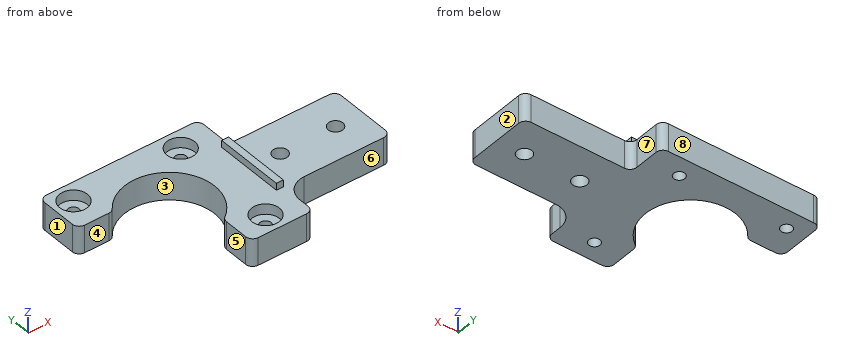
from build123d import *

# Parameters (mm, degrees)
ESQUISSE1_W             = 77
ESQUISSE1_H             = 42
BOSS_EXTRU_1_DEPTH      = 8
ESQUISSE3_R             = 4
ENL_V_MAT_EXTRU_1_DEPTH = 3
ESQUISSE4_R             = 13
ENL_V_MAT_EXTRU_2_DEPTH = 9
ESQUISSE5_W             = 28
ESQUISSE5_H             = 28
ENL_V_MAT_EXTRU_3_DEPTH = 9
ESQUISSE10_R            = 1.6
ENL_V_MAT_EXTRU_4_DEPTH = 6
ESQUISSE11_W            = 31
ESQUISSE11_H            = 11
ENL_V_MAT_EXTRU_5_DEPTH = 9
ESQUISSE12_R            = 2.1
ENL_V_MAT_EXTRU_6_DEPTH = 9
CONG_1_R                = 6
CONG_2_R                = 2
SKETCH1_W               = 2
SKETCH1_H               = 20
BOSS_EXTRUDE1_DEPTH     = 2


with BuildPart() as part:
    # Esquisse1 → Boss.-Extru.1 (new body)
    with BuildSketch(Plane.XY):
        with Locations((38.5, 21)):
            Rectangle(ESQUISSE1_W, ESQUISSE1_H)
    extrude(amount=BOSS_EXTRU_1_DEPTH)

    # Esquisse3 → Enlèv. mat.-Extru.1 (cut)
    with BuildSketch(Plane.XY.offset(8)):
        with Locations((5.5, 36.5)):
            Circle(ESQUISSE3_R)
        with Locations((36.5, 36.5)):
            Circle(ESQUISSE3_R)
        with Locations((36.5, 5.5)):
            Circle(ESQUISSE3_R)
    extrude(amount=-ENL_V_MAT_EXTRU_1_DEPTH, mode=Mode.SUBTRACT)

    # Esquisse4 → Enlèv. mat.-Extru.2 (cut, through all)
    with BuildSketch(Plane.XY.offset(8)):
        with Locations((21, 21)):
            Circle(ESQUISSE4_R)
    extrude(amount=-ENL_V_MAT_EXTRU_2_DEPTH, mode=Mode.SUBTRACT)

    # Esquisse5 → Enlèv. mat.-Extru.3 (cut, through all)
    with BuildSketch(Plane.XY.offset(8)):
        with Locations((14, 14)):
            Rectangle(ESQUISSE5_W, ESQUISSE5_H)
    extrude(amount=-ENL_V_MAT_EXTRU_3_DEPTH, mode=Mode.SUBTRACT)

    # Esquisse10 → Enlèv. mat.-Extru.4 (cut, through all)
    with BuildSketch(Plane.XY.offset(5)):
        with Locations((5.5, 36.5)):
            Circle(ESQUISSE10_R)
        with Locations((36.5, 36.5)):
            Circle(ESQUISSE10_R)
        with Locations((36.5, 5.5)):
            Circle(ESQUISSE10_R)
    extrude(amount=-ENL_V_MAT_EXTRU_4_DEPTH, mode=Mode.SUBTRACT)

    # Esquisse11 → Enlèv. mat.-Extru.5 (cut, through all)
    with BuildSketch(Plane.XY.offset(8)):
        with Locations((61.5, 5.5)):
            Rectangle(ESQUISSE11_W, ESQUISSE11_H)
        with Locations((61.5, 36.5)):
            Rectangle(ESQUISSE11_W, ESQUISSE11_H)
    extrude(amount=-ENL_V_MAT_EXTRU_5_DEPTH, mode=Mode.SUBTRACT)

    # Esquisse12 → Enlèv. mat.-Extru.6 (cut, through all)
    with BuildSketch(Plane.XY.offset(8)):
        with Locations((53, 21)):
            Circle(ESQUISSE12_R)
        with Locations((69, 21)):
            Circle(ESQUISSE12_R)
    extrude(amount=-ENL_V_MAT_EXTRU_6_DEPTH, mode=Mode.SUBTRACT)

    # Congé1
    cong_1_edges = [part.edges().sort_by_distance(p)[0] for p in [
        (46, 11, 4),
    ]]
    fillet(cong_1_edges, radius=CONG_1_R)

    # Congé2
    cong_2_edges = [part.edges().sort_by_distance(p)[0] for p in [
        (28, 10.04554885, 4),
        (10.04554885, 28, 4),
        (0, 28, 4),
        (28, 0, 4),
        (77, 11, 4),
        (46, 0, 4),
        (0, 42, 4),
        (77, 31, 4),
        (46, 31, 4),
        (46, 42, 4),
    ]]
    fillet(cong_2_edges, radius=CONG_2_R)

    # Sketch1 → Boss-Extrude1 (add)
    with BuildSketch(Plane.XY.offset(8)):
        with Locations((45, 21)):
            Rectangle(SKETCH1_W, SKETCH1_H)
    extrude(amount=BOSS_EXTRUDE1_DEPTH)


solid = part.part
Can you work these out from the model? Positions are in its coordinate system, mm. Face numbers are marked on the shaded views. A direction names the side the tool comes from. Coordinates: 2 decimals unless noted, no trailing zeros. Order: outer loops, then holes, each group sorted by start corner. A loop starts at its lowest first (then second) coordinate and runs counter-clockwise, first axis right, second up. Notation, with made-up numbers: M -3,13 L 12,13 A16 ccw 12,26 Z; hole C 56.5,71.25 d11. An arc over 180 degrees is marked long. Write item = value, one per line.
(1) If we mould it in two halves opening along X, with no side actions, what happens to the marked faces 1, 2, 3 and 4? For each: pulls with the +X half, pulls with the -X half, needs draft (parallel to the pull), parting line crosses it, or undercut.
Results are:
face_1 = pulls with the -X half
face_2 = pulls with the +X half
face_3 = undercut
face_4 = needs draft
(2) For pin 1 Ø3.5 at (y, z) = (3, 5) entering from +X; pin 2 Ø6 at (y, z) = (4.5, 7.5) entering from +X; pin 3 Ø23.5 at (x, y) = (21, 21) entering from +Z; pin 4 Ø5.5 at (y, z) = (6, 5.5) entering from -X, each with a flat end and sliding along its axis, tell me the tip position at first contact or that it passes through.
Results are:
pin_1 = 46
pin_2 = 46.55
pin_3 = through
pin_4 = 28
(3) Suppose I cut it at B-B on x = 69. Please give me the cut outline in (y, z).
Results are:
outline = M 11,0 L 18.9,0 L 18.9,8 L 11,8 Z; M 23.1,0 L 31,0 L 31,8 L 23.1,8 Z
(4) Suppose I cut it at A-A on y = 36.5. Please give me the cut outline in (x, z).
Results are:
outline = M 0,0 L 3.9,0 L 3.9,5 L 1.5,5 L 1.5,8 L 0,8 Z; M 7.1,0 L 34.9,0 L 34.9,5 L 32.5,5 L 32.5,8 L 9.5,8 L 9.5,5 L 7.1,5 Z; M 38.1,0 L 46,0 L 46,8 L 40.5,8 L 40.5,5 L 38.1,5 Z
(5) Suppose I cut it at D-D on x = 36.5. Please give me the cut outline in (y, z), plus the area to 3 significant figures.
Results are:
outline = M 0,0 L 3.9,0 L 3.9,5 L 1.5,5 L 1.5,8 L 0,8 Z; M 7.1,0 L 34.9,0 L 34.9,5 L 32.5,5 L 32.5,8 L 9.5,8 L 9.5,5 L 7.1,5 Z; M 38.1,0 L 42,0 L 42,8 L 40.5,8 L 40.5,5 L 38.1,5 Z
area = 256 mm2
(6) Suppose I cut it at C-C on z = 2.75. Please give me the cut outline in (x, y).
Results are:
outline = M 0,30 A2 ccw 2,28 L 9,28 A2 ccw 10.6,28.8 A13 cw long 28.8,10.6 A2 ccw 28,9 L 28,2 A2 ccw 30,0 L 44,0 A2 ccw 46,2 L 46,5 A6 cw 52,11 L 75,11 A2 ccw 77,13 L 77,29 A2 ccw 75,31 L 48,31 A2 cw 46,33 L 46,40 A2 ccw 44,42 L 2,42 A2 ccw 0,40 Z; hole C 5.5,36.5 d3.2; hole C 36.5,5.5 d3.2; hole C 36.5,36.5 d3.2; hole C 53,21 d4.2; hole C 69,21 d4.2
(7) I need wall thicknesses on line 1 along Y through (x, z) = (53, 5.25); line 2 along Y through (x, z) = (35, 6); line 3 along Y through (x, z) = (5.5, 7.2). Which ranges of each line are inside material? Lowest first, please. Write a range as [from, to].
Results are:
line_1 = [11, 18.9], [23.1, 31]
line_2 = [0, 1.79], [9.21, 32.79], [40.21, 42]
line_3 = [28, 32.5], [40.5, 42]
(8) For the marked faces 5, 6, 7 and 8, which set-ups out of +Z, -Z, +X, -X, +Y, -Y let a thin tool reach every point of the face, with its end or its side?
Results are:
face_5 = +Z, -Z, -X, -Y
face_6 = +Z, -Z, +X, -Y
face_7 = +Z, -Z, +X, +Y
face_8 = +Z, -Z, +X, -X, +Y
